Input: part model. Units: mm. Frame: model coordinates. A direction names the side the tool comes from. Round coordinates to 2 decimals unless told otherwise and drop trailing zeros. Order: outer loops, then holes, each group sorted by start corner. A loop starts at its lowest first (then second) coordinate and runs counter-clockwise, first axis right, second up. Notation, with made-up numbers: (67, -3.5) - (72, -3.5) arc R25 ccw to (72, 19.5) - close; hole circle Ø3 at (19.25, 30). An arc over 180 degrees is marked (long way). One line per item, written item: value. Start each with the question number.
from build123d import *

# Parameters (mm, degrees)
SKETCH1_W           = 12.7
SKETCH1_H           = 50.8
BOSS_EXTRUDE1_DEPTH = 12.7
SKETCH2_W           = 12.7
SKETCH2_H           = 6.35
SKETCH2_H_2         = 5.842
BOSS_EXTRUDE2_DEPTH = 34.925
SKETCH4_R           = 6.35
BOSS_EXTRUDE3_DEPTH = 6.985
CUT_EXTRUDE1_START  = -3.937
CUT_EXTRUDE1_DEPTH  = 3.937
CUT_EXTRUDE2_DEPTH  = 12.827
BOSS_EXTRUDE4_START = -12.7
SKETCH6_W           = 38.1
SKETCH6_H           = 12.7
BOSS_EXTRUDE4_DEPTH = 88.9
SKETCH7_W           = 22.86
SKETCH7_H           = 12.7
CUT_EXTRUDE3_DEPTH  = 7.112
SKETCH9_W           = 2.794
SKETCH9_H           = 12.7
CUT_EXTRUDE4_DEPTH  = 91.628182394


with BuildPart() as part:
    # Sketch1 → Boss-Extrude1 (new body)
    with BuildSketch(Plane.XY):
        Rectangle(SKETCH1_W, SKETCH1_H)
    extrude(amount=BOSS_EXTRUDE1_DEPTH)

    # Sketch2 → Boss-Extrude2 (add)
    with BuildSketch(Plane.XY.offset(12.7)):
        with Locations((0, 22.225)):
            Rectangle(SKETCH2_W, SKETCH2_H)
        with Locations((0, 9.144)):
            Rectangle(SKETCH2_W, SKETCH2_H_2)
    extrude(amount=BOSS_EXTRUDE2_DEPTH)

    # Sketch4 → Boss-Extrude3 (add)
    with BuildSketch(Plane(origin=(0, 12.065, 0), x_dir=(1, 0, 0), z_dir=(0, 1, 0))):
        with Locations((0, -41.275)):
            Circle(SKETCH4_R)
    extrude(amount=BOSS_EXTRUDE3_DEPTH)

    # Sketch5 → Cut-Extrude1 (cut)
    with BuildSketch(Plane.XZ.offset(-6.223).offset(CUT_EXTRUDE1_START)):
        with BuildLine():
            Line((3.8, 16.775), (3.8, 30.925))
            ThreePointArc((3.8, 30.925), (4.31316702, 34.08727766), (5.8, 36.925))
            ThreePointArc((5.8, 36.925), (6.08989801, 37.34109072), (6.35, 37.776428863))
            Line((6.35, 37.776428863), (6.35, 41.275))
            ThreePointArc((6.35, 41.275), (4.490128061, 45.765128061), (0, 47.625))
            ThreePointArc((0, 47.625), (-4.490128061, 45.765128061), (-6.35, 41.275))
            Line((-6.35, 41.275), (-6.35, 37.776428863))
            ThreePointArc((-6.35, 37.776428863), (-6.08989801, 37.34109072), (-5.8, 36.925))
            ThreePointArc((-5.8, 36.925), (-4.313167019, 34.08727766), (-3.8, 30.925))
            Line((-3.8, 30.925), (-3.8, 16.775))
            ThreePointArc((-3.8, 16.775), (0, 12.975), (3.8, 16.775))
        make_face()
        with BuildLine():
            ThreePointArc((-6.35, 41.275), (-4.490128061, 45.765128061), (0, 47.625))
            Line((0, 47.625), (-3.498571137, 47.625))
            Line((-3.498571137, 47.625), (-6.35, 47.625))
            Line((-6.35, 47.625), (-6.35, 44.773571137))
            Line((-6.35, 44.773571137), (-6.35, 41.275))
        make_face()
        with BuildLine():
            ThreePointArc((0, 47.625), (4.490128061, 45.765128061), (6.35, 41.275))
            Line((6.35, 41.275), (6.35, 44.773571137))
            Line((6.35, 44.773571137), (6.35, 47.625))
            Line((6.35, 47.625), (3.498571137, 47.625))
            Line((3.498571137, 47.625), (0, 47.625))
        make_face()
    extrude(amount=CUT_EXTRUDE1_DEPTH, mode=Mode.SUBTRACT)

    # Sketch5<3> → Cut-Extrude2 (cut)
    with BuildSketch(Plane.XZ.offset(-6.223)):
        with BuildLine():
            ThreePointArc((-6.35, 41.275), (-4.490128061, 45.765128061), (0, 47.625))
            Line((0, 47.625), (-3.498571137, 47.625))
            Line((-3.498571137, 47.625), (-6.35, 47.625))
            Line((-6.35, 47.625), (-6.35, 44.773571137))
            Line((-6.35, 44.773571137), (-6.35, 41.275))
        make_face()
        with BuildLine():
            ThreePointArc((0, 47.625), (4.490128061, 45.765128061), (6.35, 41.275))
            Line((6.35, 41.275), (6.35, 44.773571137))
            Line((6.35, 44.773571137), (6.35, 47.625))
            Line((6.35, 47.625), (3.498571137, 47.625))
            Line((3.498571137, 47.625), (0, 47.625))
        make_face()
    extrude(amount=-CUT_EXTRUDE2_DEPTH, mode=Mode.SUBTRACT)

    # Sketch6 → Boss-Extrude4 (add)
    with BuildSketch(Plane(origin=(0, 0, 0), x_dir=(-1, 0, 0), z_dir=(0, 0, -1)).offset(BOSS_EXTRUDE4_START)):
        with Locations((0, -19.05)):
            Rectangle(SKETCH6_W, SKETCH6_H)
    extrude(amount=BOSS_EXTRUDE4_DEPTH)

    # Sketch7 → Cut-Extrude3 (cut)
    with BuildSketch(Plane(origin=(0, -12.7, 0), x_dir=(1, 0, 0), z_dir=(0, 1, 0))):
        with Locations((-0.254, 67.31)):
            Rectangle(SKETCH7_W, SKETCH7_H)
    extrude(amount=-CUT_EXTRUDE3_DEPTH, mode=Mode.SUBTRACT)

    # Sketch9 → Cut-Extrude4 (cut, through all)
    with BuildSketch(Plane(origin=(0, -19.812, 0), x_dir=(1, 0, 0), z_dir=(0, 1, 0))):
        with Locations((5.334, 67.31)):
            Rectangle(SKETCH9_W, SKETCH9_H)
    extrude(amount=-CUT_EXTRUDE4_DEPTH, mode=Mode.SUBTRACT)


solid = part.part
1. Section C-C (y = 14). Return the cut outline in (x, z) (3 decimals).
2. Pin query (flat end, axial travel): pin 1 (4 mm diameter, centred on x = -1, z = 32.5, fed in from -Y); pin 2 (10 mm diameter, centred on x = -1, z = -70, fed in from +Y); pin 3 (1.3 mm diameter, centred on x = 8.5, z = -69, fed in from +Y). Return the tip coordinate at first contact, or that it passes through.
3. Set-up query: faces 1 (the face through (6.35, 10, 13)), 2 (the face through (0, 7, 0)), 3 (the face through (0, 10.16, 31)), 4 (the face through (6.731, -23, -67)), 5 (the face through (0, -13, 12.7)). Return all of +Z, -Z, +X, -X, +Y, -Y with unobstructed straight access to the full face (end or side cutting, diameter ignored); none if empty.
4. Section D-D (x = 8.5). Return the cut outline in (y, z).
5. Section A-A (z = 21). Return the cut outline in (x, y) (3 decimals).
6. Pull-direction query (X, two-part tool) for faces 6 (the face through (11.176, -16, -67)), 7 (the face through (-6.35, 10, 13)), 8 (the face through (0, -25.4, -31)), 9 (the face through (-4, -19.812, -67)); classes: released by +X, released by -X, zero draft, split by the parting line, or undercut.
7. Line query: line 1 (Z direction, x = 11, y = -15.5); line 2 (Z direction, x = -6, y = -5.5); line 3 (Y direction, x = -2, z = -41). Output: solid intervals per line, ascending. Write a range as from..to.
8. Section B-B (y = -18.5). Return the cut outline in (x, z), then the cut area to 3 significant figures.
Solved:
1. outline: (-6.35, 0) - (6.35, 0) - (6.35, 12.7) - (-6.35, 12.7) - close; circle Ø12.7 at (0, 41.275)
2. pin 1: stops at y = 10.16
2. pin 2: stops at y = -12.7
2. pin 3: stops at y = -19.81
3. face 1: +Z, -Z, +X, +Y
3. face 2: -Z, +X, -X, +Y
3. face 3: +Z, -Y
3. face 4: +Y, -Y
3. face 5: +Z, +X, -X, -Y
4. outline: (-25.4, -76.2) - (-12.7, -76.2) - (-12.7, -73.66) - (-19.81, -73.66) - (-19.81, -60.96) - (-12.7, -60.96) - (-12.7, 12.7) - (-25.4, 12.7) - close
5. outline: (-6.35, 6.223) - (-3.8, 6.223) - (-3.8, 10.16) - (3.8, 10.16) - (3.8, 6.223) - (6.35, 6.223) - (6.35, 12.065) - (-6.35, 12.065) - close; (-6.35, 19.05) - (6.35, 19.05) - (6.35, 25.4) - (-6.35, 25.4) - close
6. face 6: undercut
6. face 7: released by -X
6. face 8: zero draft
6. face 9: undercut
7. line 1: z = -76.2..-73.66, -60.96..12.7
7. line 2: z = 0..12.7
7. line 3: y = -25.4..-12.7
8. outline: (-19.05, -76.2) - (19.05, -76.2) - (19.05, 12.7) - (-19.05, 12.7) - close; hole (-11.68, -73.66) - (11.18, -73.66) - (11.18, -60.96) - (-11.68, -60.96) - close
8. area: 3,100 mm²
